Geometry check sheet. Reference: drawing and pictorial views, mm from the part's lowest x, y, z. Coordinates: 2 decimals unless noted, no trailing zeros. Write each loop counter-clockwise with the first axis right and the second up, starting at its lowest first coordinate (ties: lowest second). Pieces come first, ordered by that corner, then holes. Notation, with made-up numbers: (-16, 36) -> (33, 36) arc R14 cw to (33, 50) -> close; hole circle Ø3 at (44, 24). An arc over 180 degrees is marked (long way). Use a Markdown table: item, result.
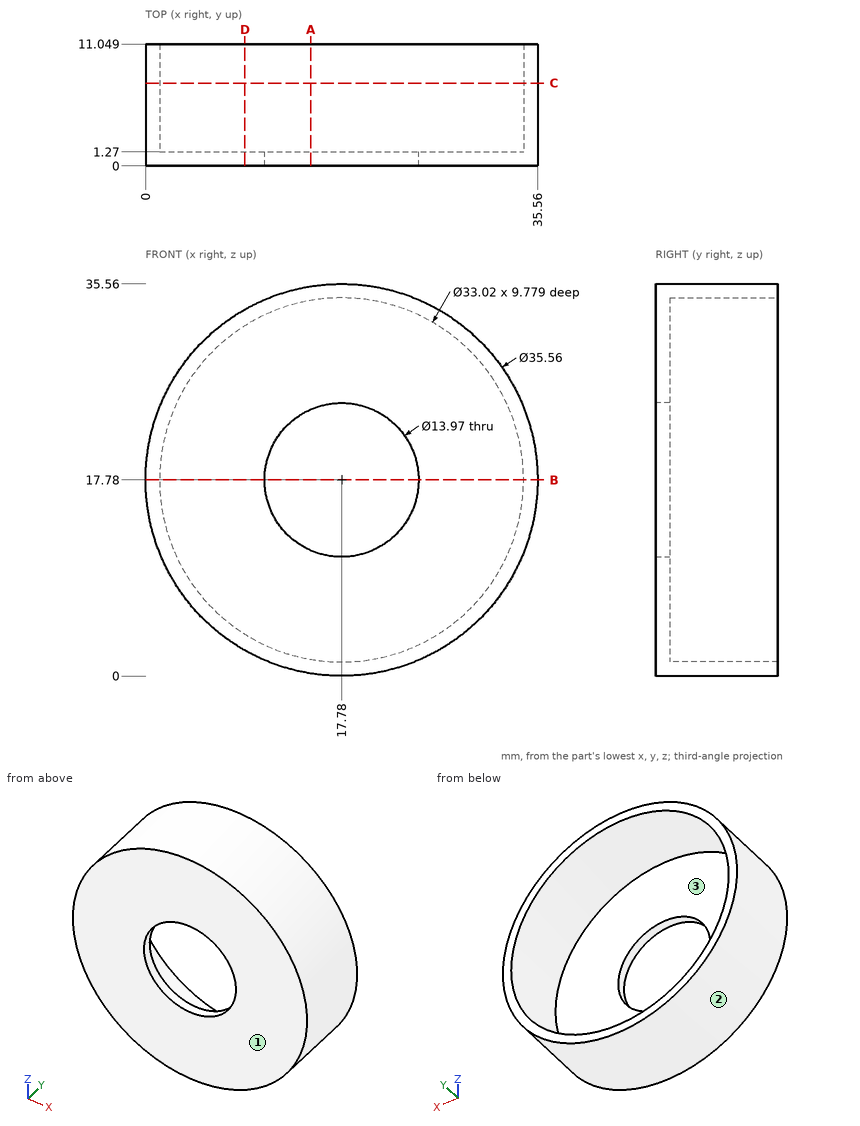
Item 1: Section check A-A on x = 15. Record the boundary of the cut face in (y, z), then the cut area to 3 significant figures.
Answer block:
| item | result |
|---|---|
| outline | (0, 0.22) -> (11.05, 0.22) -> (11.05, 1.51) -> (1.27, 1.51) -> (1.27, 11.37) -> (0, 11.37) -> close; (0, 24.19) -> (1.27, 24.19) -> (1.27, 34.05) -> (11.05, 34.05) -> (11.05, 35.34) -> (0, 35.34) -> close |
| area | 53.5 mm^2 |
Item 2: Section check D-D on x = 9. Record the boundary of the cut face in (y, z).
Answer block:
| item | result |
|---|---|
| outline | (0, 2.32) -> (11.05, 2.32) -> (11.05, 3.8) -> (1.27, 3.8) -> (1.27, 31.76) -> (11.05, 31.76) -> (11.05, 33.24) -> (0, 33.24) -> close |
Item 3: Thickness scan on L1, parallel to X at y = 0.95, z = 17.78 (3 decimals); L2, parallel to X at y = 5, z = 17.78; L3, parallel to Y at x = 24, z = 12. Record the ranges inside material, lowest first. Write a range as [from, to].
Answer block:
| item | result |
|---|---|
| L1 | x = [0, 10.795], [24.765, 35.56] |
| L2 | x = [0, 1.27], [34.29, 35.56] |
| L3 | y = [0, 1.27] |
Item 4: Section check B-B on z = 17.78. Record the boundary of the cut face in (x, y) (3 decimals), then the cut area to 3 significant figures.
Answer block:
| item | result |
|---|---|
| outline | (0, 0) -> (10.795, 0) -> (10.795, 1.27) -> (1.27, 1.27) -> (1.27, 11.049) -> (0, 11.049) -> close; (24.765, 0) -> (35.56, 0) -> (35.56, 11.049) -> (34.29, 11.049) -> (34.29, 1.27) -> (24.765, 1.27) -> close |
| area | 52.3 mm^2 |
Item 5: Section check C-C on y = 7.5. Record the boundary of the cut face in (x, z).
Answer block:
| item | result |
|---|---|
| outline | circle Ø35.56 at (17.78, 17.78); hole circle Ø33.02 at (17.78, 17.78) |
Item 6: Mould release check, pull along X, two halves, no side actions. Record for the marked faces 1, 2 and 3: +X half, -X half, draft (parallel to the pull), parting line (faces both ways), or undercut.
Answer block:
| item | result |
|---|---|
| face 1 | draft |
| face 2 | parting line |
| face 3 | undercut |
Item 7: Depth check by flat-ended pin: P1, Ø1.5, axis at x = 29, y = 7.5, coming from the +Z side; P2, Ø5, axis at x = 25, y = 3, coming from the +Z side; P3, Ø2, axis at x = 4.5, y = 4.5, coming from the -Z side. Enter the tip coordinate at first touch or a pass-through.
Answer block:
| item | result |
|---|---|
| P1 | stops at z = 32.15 |
| P2 | stops at z = 34.92 |
| P3 | stops at z = 4.92 |
